from build123d import *

# Parameters (mm, degrees)
SZKIC1_R                    = 11
SZKIC1_R_2                  = 1.25
DODANIE_WYCI_GNI_CIE1_DEPTH = 2
SFAZOWANIE1_SIZE            = 0.3
SFAZOWANIE2_SIZE            = 2


with BuildPart() as part:
    # Szkic1 → Dodanie-wyciągnięcie1 (new body)
    with BuildSketch(Plane.XY):
        with BuildLine():
            Line((-27, -20), (27, -20))
            ThreePointArc((27, -20), (29.121320344, -19.121320344), (30, -17))
            Line((30, -17), (30, 17))
            ThreePointArc((30, 17), (29.121320344, 19.121320344), (27, 20))
            Line((27, 20), (-27, 20))
            ThreePointArc((-27, 20), (-29.121320344, 19.121320344), (-30, 17))
            Line((-30, 17), (-30, -17))
            ThreePointArc((-30, -17), (-29.121320344, -19.121320344), (-27, -20))
        make_face()
        Circle(SZKIC1_R, mode=Mode.SUBTRACT)
        with Locations((-22, 14.666666667)):
            Circle(SZKIC1_R_2, mode=Mode.SUBTRACT)
        with Locations((22, 14.666666667)):
            Circle(SZKIC1_R_2, mode=Mode.SUBTRACT)
        with Locations((22, -14.666666667)):
            Circle(SZKIC1_R_2, mode=Mode.SUBTRACT)
        with Locations((-10.606601718, -10.606601718)):
            Circle(SZKIC1_R_2, mode=Mode.SUBTRACT)
        with Locations((10.606601718, -10.606601718)):
            Circle(SZKIC1_R_2, mode=Mode.SUBTRACT)
        with Locations((10.606601718, 10.606601718)):
            Circle(SZKIC1_R_2, mode=Mode.SUBTRACT)
        with Locations((-10.606601718, 10.606601718)):
            Circle(SZKIC1_R_2, mode=Mode.SUBTRACT)
        with Locations((-22, -14.666666667)):
            Circle(SZKIC1_R_2, mode=Mode.SUBTRACT)
    extrude(amount=DODANIE_WYCI_GNI_CIE1_DEPTH)

    # Sfazowanie1
    sfazowanie1_edges = [part.edges().sort_by_distance(p)[0] for p in [
        (-11, 0, 0),
        (-11, 0, 2),
    ]]
    chamfer(sfazowanie1_edges, length=SFAZOWANIE1_SIZE)

    # Sfazowanie2
    sfazowanie2_edges = [part.edges().sort_by_distance(p)[0] for p in [
        (-11.856601718, -10.606601718, 2),
        (9.356601718, -10.606601718, 2),
        (9.356601718, 10.606601718, 2),
        (-11.856601718, 10.606601718, 2),
    ]]
    chamfer(sfazowanie2_edges, length=SFAZOWANIE2_SIZE - 0.0001)  # a hair under: the kernel refuses the full size


solid = part.part
For this review, take the finished solid that the model builds, in its own axes (mm). Give positions to 0.01 mm unless a question says otherwise; leave off trailing zeros. Loops run counter-clockwise (first coordinate to the right, second up) from the corner with the lowest first, then second, coordinate; pieces in that order, holes last. Notation, with made-up numbers: M -8.75,-33.5 L 35.25,-33.5 A21 cw 35.25,-5.5 Z; hole C 31,-9.5 d2. An arc over 180 degrees is marked long. Put each result on its own line as item: value. Start each with the question number.
(1) For pin 1 (8 mm diameter, centred on x = 16, y = 14, fed in from -Z); pin 2 (3 mm diameter, centred on x = -10.61, y = -10.61, fed in from +Z), all flat-tipped, find the tip position at first contact; note any pin that passes through.
(2) Add section D-D, the plane x = 0. Write out the cut boundary in (y, z), then the cut area to 3 significant figures.
(3) Add section A-A, the plane y = 0. Write out the cut boundary in (x, z).
(4) The part is to be moulded in two halves that separate along X. For faces 1 (the flat face through (-7.1, 9.2, 0)), 2 (the cylindrical face through (-2.38, -10.74, 0.99)), 3 (the cylindrical face through (23.155, -15.145, 0.986)), 4 (the cylindrical face through (-29.14, -19.1, 0.99)), say which applies: +X half, -X half, draft (parallel to the pull), parting line (faces both ways), or undercut.
(5) Wall thickness on L1, parallel to Y at x = -22, z = 0.75; L2, parallel to Y at x = 9, z = 1.15; L3, parallel to Y at x = 9.5, z = 0.8: over which ranges is each line inside the solid? List them lowest first.
(6) Add section B-B, the plane x = 22. Write out the cut boundary in (y, z).
(7) Add section C-C, the plane z = 0.7. Give the number of separate pieces and of enclosed holes in the cut face, then the cut area to 3 significant figures.
Result:
1. pin 1: stops at z = 0
1. pin 2: stops at z = 0.25
2. outline: M -20,0 L -11.3,0 L -11,0.3 L -11,1.7 L -11.3,2 L -20,2 Z; M 11,0.3 L 11.3,0 L 20,0 L 20,2 L 11.3,2 L 11,1.7 Z
2. area: 35.8 mm^2
3. outline: M -30,0 L -11.3,0 L -11,0.3 L -11,1.7 L -11.3,2 L -30,2 Z; M 11,0.3 L 11.3,0 L 30,0 L 30,2 L 11.3,2 L 11,1.7 Z
4. face 1: draft
4. face 2: undercut
4. face 3: undercut
4. face 4: -X half
5. L1: y = -20 to -15.92, -13.42 to 13.42, 15.92 to 20
5. L2: y = -20 to -12.39, -8.82 to -6.32, 6.32 to 8.82, 12.39 to 20
5. L3: y = -20 to -12.33, -8.88 to -5.55, 5.55 to 8.88, 12.33 to 20
6. outline: M -20,0 L -15.92,0 L -15.92,2 L -20,2 Z; M -13.42,0 L 13.42,0 L 13.42,2 L -13.42,2 Z; M 15.92,0 L 20,0 L 20,2 L 15.92,2 Z
7. separate pieces: 1
7. enclosed holes: 9
7. area: 1,940 mm^2
